from build123d import *

# Parameters (mm, degrees)
F_1_8_0_1250_DOWEL_HOLE1_D = 3.175
CIRPATTERN2_COUNT          = 3
CUT_EXTRUDE1_START         = -10
SKETCH7_R                  = 15.875
CUT_EXTRUDE1_DEPTH         = 10
FILLET1_R                  = 6.35
BOSS_EXTRUDE1_START        = 3.175
SKETCH11_R                 = 3.1623
SKETCH11_R_2               = 2.0193
BOSS_EXTRUDE1_DEPTH        = 3.175


with BuildPart() as part:
    # Sketch1 → Revolve1 (revolve)
    with BuildSketch(Plane(origin=(0, 0, 0), x_dir=(0, 0, -1), z_dir=(1, 0, 0)), mode=Mode.PRIVATE) as revolve1_sk:
        Polygon((0, 2.0193), (0, 4.318), (5.08, 4.318), (5.08, 15.875), (8.255, 15.875), (8.255, 2.0193), align=None)
    revolve(revolve1_sk.sketch.rotate(Axis((0, 0, 0), (0, 0, -1)), 90), axis=Axis((0, 0, 0), (0, 0, -1)))

    # 1/8 (0.1250) Dowel Hole1 (through all)
    with Locations(Plane.XY.offset(-5.08)):
        with Locations((0, 9.525), (0, 0)):
            f_1_8_0_1250_dowel_hole1 = Hole(F_1_8_0_1250_DOWEL_HOLE1_D / 2)

    # CirPattern2: 1/8 (0.1250) Dowel Hole1 ×3 about axis
    cirpattern2_axis = Axis((0, 0, 0), (0, 0, 1))
    for i in range(1, CIRPATTERN2_COUNT):
        add(f_1_8_0_1250_dowel_hole1.rotate(cirpattern2_axis, i * 360 / CIRPATTERN2_COUNT), mode=Mode.SUBTRACT)

    # Sketch7 → Cut-Extrude1 (cut)
    with BuildSketch(Plane.XY.offset(-5.08).offset(CUT_EXTRUDE1_START)):
        Circle(SKETCH7_R)
        with BuildLine():
            ThreePointArc((-4.7625, 9.525), (0, 14.2875), (4.7625, 9.525))
            Line((4.7625, 9.525), (4.7625, 2.749630657))
            Line((4.7625, 2.749630657), (10.630141971, -0.638054014))
            ThreePointArc((10.630141971, -0.638054014), (12.373337957, -7.14375), (5.867641971, -8.886945986))
            Line((5.867641971, -8.886945986), (0, -5.499261314))
            Line((0, -5.499261314), (-5.867641971, -8.886945986))
            ThreePointArc((-5.867641971, -8.886945986), (-12.373337957, -7.14375), (-10.630141971, -0.638054014))
            Line((-10.630141971, -0.638054014), (-4.7625, 2.749630657))
            Line((-4.7625, 2.749630657), (-4.7625, 9.525))
        make_face(mode=Mode.SUBTRACT)
    extrude(amount=CUT_EXTRUDE1_DEPTH, mode=Mode.SUBTRACT)

    # Fillet1
    fillet1_edges = [part.edges().sort_by_distance(p)[0] for p in [
        (0, -5.499261314, -6.6675),
        (4.7625, 2.749630657, -6.6675),
        (-4.7625, 2.749630657, -6.6675),
    ]]
    fillet(fillet1_edges, radius=FILLET1_R)

    # Sketch11 → Boss-Extrude1 (add)
    with BuildSketch(Plane.XY.offset(BOSS_EXTRUDE1_START)):
        with Locations(Location((0, 0, 0), (0, 0, 180))):
            Circle(SKETCH11_R)
        Circle(SKETCH11_R_2, mode=Mode.SUBTRACT)
    extrude(amount=-BOSS_EXTRUDE1_DEPTH)


solid = part.part
Could you check a few things on this model? Use its own coordinates, in mm. A direction names the side the tool comes from. Coordinates: 2 decimals unless noted, no trailing zeros. Write each loop counter-clockwise with the first axis right and the second up, starting at its lowest first coordinate (ties: lowest second). Pieces come first, ordered by that corner, then holes. Notation, with made-up numbers: (52.5, 41.25) - (57.5, 41.25) arc R11 cw to (57.5, 45.25) - close; hole circle Ø8 at (56, 57). An arc over 180 degrees is marked (long way). Put each result on its own line as item: value. Start each with the question number.
Q1. I'm going to push flat-ended pins straight in: P1, Ø2.5, axis at x = 0, y = 9.525, coming from the -Z side; P2, Ø5.5, axis at x = 0, y = 0, coming from the +Z side (3 decimals); P3, Ø8, axis at x = 8.5, y = 11, coming from the +Z side; P4, Ø2.5, axis at y = 8, z = -6.5, coming from the -X side. Where does each tip first touch, or does it pass through?
Q2. Which directions (+Z, -Z, +X, -X, +Y, -Y) give clear straight access to the entire face, cutting with the end or side of a thin tool? Please do faces 1 (the cylindrical face through (-0.56, -4.28, -2.58)), 2 (the flat face through (4.762, 8, -7)), 3 (the flat face through (-4.762, 8, -7)).
Q3. I want a section at C-C on x = -9. Write out the boundary of the cut face in (y, z) (3 decimals), plus the area to 3 significant figures.
Q4. I want a section at B-B on x = 0. Write out the boundary of the cut face in (y, z) (1 decimal), plus the area to 3 significant figures.
Q5. Thinking about a two-plate mould opening in Y: for faces 4 (the cylindrical face through (1, 3, 2)), 5 (the flat face through (0, 5, -5.08)), 6 (the cylindrical face through (7.516, -6.171, -6.69)), 7 (the cylindrical face through (-6.663, -4.693, -6.69)), which applies, pulls with the +Y half, pulls with the -Y half, needs draft (parallel to the pull), parting line crosses it, or undercut?
Q6. I want a section at D-D on z = -7.5. Count the separate pieces of the cut face and the enclosed holes in it, plus the area to 3 significant figures.
Q7. Please list where these lines run through material, in increasing order: L1, parallel to Y at x = 0, z = -4.25; L2, parallel to Y at x = 0, z = 1.7; L3, parallel to X at y = 0.25, z = -4.5.
Q8. I want a section at A-A on y = 0. Write out the boundary of the cut face in (x, z) (3 decimals).
Checks:
1. P1: through
1. P2: z = 3.175
1. P3: z = -5.08
1. P4: x = -4.76
2. face 1: +Z
2. face 2: +Z, -Z, +X, +Y
2. face 3: +Z, -Z, -X, +Y
3. outline: (-9.465, -8.255) - (-6.161, -8.255) - (-6.161, -5.08) - (-9.465, -5.08) - close; (-3.364, -8.255) - (0.303, -8.255) - (0.303, -5.08) - (-3.364, -5.08) - close
3. area: 22.1 mm²
4. outline: (-6.5, -8.3) - (-2, -8.3) - (-2, 3.2) - (-3.2, 3.2) - (-3.2, 0) - (-4.3, 0) - (-4.3, -5.1) - (-6.5, -5.1) - close; (2, -8.3) - (7.9, -8.3) - (7.9, -5.1) - (4.3, -5.1) - (4.3, 0) - (3.2, 0) - (3.2, 3.2) - (2, 3.2) - close; (11.1, -8.3) - (14.3, -8.3) - (14.3, -5.1) - (11.1, -5.1) - close
4. area: 73.7 mm²
5. face 4: parting line crosses it
5. face 5: needs draft
5. face 6: undercut
5. face 7: undercut
6. separate pieces: 1
6. enclosed holes: 4
6. area: 310 mm²
7. L1: -4.32 to -2.02, 2.02 to 4.32
7. L2: -3.16 to -2.02, 2.02 to 3.16
7. L3: -4.31 to -2, 2 to 4.31
8. outline: (-9.525, -8.255) - (-2.019, -8.255) - (-2.019, 3.175) - (-3.162, 3.175) - (-3.162, 0) - (-4.318, 0) - (-4.318, -5.08) - (-9.525, -5.08) - close; (2.019, -8.255) - (9.525, -8.255) - (9.525, -5.08) - (4.318, -5.08) - (4.318, 0) - (3.162, 0) - (3.162, 3.175) - (2.019, 3.175) - close
